```python
from build123d import *

# Parameters (mm, degrees)
SKETCH1_R           = 50
BOSS_EXTRUDE1_DEPTH = 30
SKETCH2_W           = 22.8
SKETCH2_H           = 12.4
CUT_EXTRUDE1_DEPTH  = 27
SKETCH3_W           = 4
SKETCH3_H           = 1.5
CUT_EXTRUDE2_DEPTH  = 77.811457479
SKETCH4_W           = 32.2
SKETCH4_H           = 12.4
CUT_EXTRUDE3_DEPTH  = 11
CUT_EXTRUDE6_START  = -3
SKETCH5_W           = 58.2
SKETCH5_H           = 48.4
SKETCH5_W_2         = 38.2
SKETCH5_H_2         = 18.4
CUT_EXTRUDE6_DEPTH  = 25
CUT_EXTRUDE9_START  = -3
SKETCH6_R           = 45
SKETCH6_R_2         = 22.113575547
CUT_EXTRUDE9_DEPTH  = 25


with BuildPart() as part:
    # Sketch1 → Boss-Extrude1 (new body)
    with BuildSketch(Plane(origin=(0, 0, 0), x_dir=(1, 0, 0), z_dir=(0, 1, 0))):
        with Locations(Location((0, 0, 0), (0, 0, 270))):
            Circle(SKETCH1_R)
    extrude(amount=BOSS_EXTRUDE1_DEPTH)

    # Sketch2 → Cut-Extrude1 (cut)
    with BuildSketch(Plane(origin=(0, 30, 0), x_dir=(1, 0, 0), z_dir=(0, 1, 0))):
        Rectangle(SKETCH2_W, SKETCH2_H)
    extrude(amount=-CUT_EXTRUDE1_DEPTH, mode=Mode.SUBTRACT)

    # Sketch3 → Cut-Extrude2 (cut, through all)
    with BuildSketch(Plane(origin=(0, 0, 0), x_dir=(0, 0, -1), z_dir=(1, 0, 0))):
        with Locations((0, 8.25)):
            Rectangle(SKETCH3_W, SKETCH3_H)
    extrude(amount=-CUT_EXTRUDE2_DEPTH, mode=Mode.SUBTRACT)

    # Sketch4 → Cut-Extrude3 (cut)
    with BuildSketch(Plane(origin=(0, 30, 0), x_dir=(1, 0, 0), z_dir=(0, 1, 0))):
        Rectangle(SKETCH4_W, SKETCH4_H)
    extrude(amount=-CUT_EXTRUDE3_DEPTH, mode=Mode.SUBTRACT)

    # Sketch5 → Cut-Extrude6 (cut)
    with BuildSketch(Plane(origin=(0, 30, 0), x_dir=(1, 0, 0), z_dir=(0, 1, 0)).offset(CUT_EXTRUDE6_START)):
        Rectangle(SKETCH5_W, SKETCH5_H)
        Rectangle(SKETCH5_W_2, SKETCH5_H_2, mode=Mode.SUBTRACT)
    extrude(amount=-CUT_EXTRUDE6_DEPTH, mode=Mode.SUBTRACT)

    # Sketch6 → Cut-Extrude9 (cut)
    with BuildSketch(Plane(origin=(0, 30, 0), x_dir=(1, 0, 0), z_dir=(0, 1, 0)).offset(CUT_EXTRUDE9_START)):
        with Locations(Location((0, 0, 0), (0, 0, 270))):
            Circle(SKETCH6_R)
        Circle(SKETCH6_R_2, mode=Mode.SUBTRACT)
    extrude(amount=-CUT_EXTRUDE9_DEPTH, mode=Mode.SUBTRACT)


solid = part.part
```
Work out the finished part from the listing and answer in its coordinate system (mm). A direction names the side the tool comes from. Round coordinates to 2 decimals unless told otherwise and drop trailing zeros. Loops run counter-clockwise (first coordinate to the right, second up) from the corner with the lowest first, then second, coordinate; pieces in that order, holes last.
(1) The part is cut by section A-A, the plane z = 0. Give the vertices of the cut face in (x, y).
Computed values:
outline: (-50, 0) - (50, 0) - (50, 30) - (16.1, 30) - (16.1, 19) - (11.4, 19) - (11.4, 3) - (-11.4, 3) - (-11.4, 7.5) - (-19.1, 7.5) - (-19.1, 2) - (-45, 2) - (-45, 7.5) - (-50, 7.5) - close; (-50, 9) - (-45, 9) - (-45, 27) - (-19.1, 27) - (-19.1, 9) - (-11.4, 9) - (-11.4, 19) - (-16.1, 19) - (-16.1, 30) - (-50, 30) - close; hole (19.1, 2) - (45, 2) - (45, 27) - (19.1, 27) - close
(2) The part is cut by section C-C, the plane x = -9.5. Give the vertices of the cut face in (y, z), and give its area (3 significant figures).
Computed values:
outline: (0, -49.09) - (30, -49.09) - (30, -6.2) - (3, -6.2) - (3, 6.2) - (30, 6.2) - (30, 49.09) - (0, 49.09) - close; hole (2, -43.99) - (27, -43.99) - (27, -9.2) - (2, -9.2) - close; hole (2, 9.2) - (27, 9.2) - (27, 43.99) - (2, 43.99) - close
area: 871 mm2
(3) The mould has two halves that part along X. Classify faces 6 (the cylindrical face through (15.02, 14.79, 47.69)), 7 (the flat face through (-47, 7.5, 0)), 8 (the flat face through (0.6, 27, 9.4)): pulls with the +X half, pulls with the -X half, needs draft (parallel to the pull), parting line crosses it, or undercut.
Computed values:
face 6: parting line crosses it
face 7: needs draft
face 8: undercut
(4) Each of these flat-tipped pins is pushed along its axis until it touches: P1, Ø5.5, axis at y = 24, z = 2, coming from the +X side; P2, Ø12.5, axis at x = 6, y = 13.5, coming from the +Z side; P3, Ø8, axis at x = 6.5, y = 12.5, coming from the +Z side; P4, Ø1.6, axis at x = -16.5, y = 8, coming from the +Z side. Where does it stop, or does it pass through?
Computed values:
P1: stops at x = 50
P2: stops at z = 50
P3: stops at z = 49.94
P4: stops at z = 47.47
(5) The part is cut by section B-B, the plane y = 14. Give the vertices of the cut face in (x, z).
Computed values:
outline: circle Ø100 at (0, 0); (-19.1, -9.2) - (19.1, -9.2) - (19.1, 9.2) - (-19.1, 9.2) - close; hole circle Ø90 at (0, 0); hole (-11.4, -6.2) - (11.4, -6.2) - (11.4, 6.2) - (-11.4, 6.2) - close
(6) For faces 1 (the flat face through (1, 30, 10)), 2 (the flat face through (0, 3, 0)), 3 (the flat face through (1, 0, -1)), 4 (the flat face through (0, 15, -9.2)), 5 (the flat face through (-47, 9, 0)), determine the directions among +Z, -Z, +X, -X, +Y, -Y from which every point of the face is accessible in a straight line to the end or side of a thin tool.
Computed values:
face 1: +Z, -Z, +X, -X, +Y
face 2: +Y
face 3: +Z, -Z, +X, -X, -Y
face 4: none
face 5: -X
(7) The part is cut by section D-D, the plane z = -43.5. Give the vertices of the cut face in (x, y), and give its area (3 significant figures).
Computed values:
outline: (-24.65, 0) - (24.65, 0) - (24.65, 30) - (-24.65, 30) - close; hole (-11.52, 2) - (11.52, 2) - (11.52, 27) - (-11.52, 27) - close
area: 903 mm2
(8) Find the intervals of material crossed by L1, parallel to X at y = 21.75, z = 0; L2, parallel to X at y = 18, z = 0; L3, parallel to Y at x = -21.5, z = 24, in increasing order.
Computed values:
L1: x = -50 to -45, -19.1 to -16.1, 16.1 to 19.1, 45 to 50
L2: x = -50 to -45, -19.1 to -11.4, 11.4 to 19.1, 45 to 50
L3: y = 0 to 2, 27 to 30
